```python
from build123d import *

# Parameters (mm, degrees)
F0_W          = 60.96
F0_H          = 91.44
F0_W_2        = 50.8
F0_H_2        = 86.614
F1_DEPTH      = 28.448
F3_DEPTH      = 25.4
F4_W          = 66.649839282
F4_H          = 6.9823637605
F5_DEPTH      = 3.048
F6_W          = 64.9686481762
F6_H          = 4.777956934
F7_DEPTH      = 3.048
F9_DEPTH      = 2.286
F10_W         = 99.848318845
F10_H         = 48.2080141082
F11_DEPTH     = 50.8
F13_T1_DEPTH  = 15.8581495789
F13_T3_DEPTH  = 15.8581495789
F13_T8_DEPTH  = 41.5121495789
F13_T13_DEPTH = 41.5121495789
F13_T18_DEPTH = 41.5121495789
F13_T23_DEPTH = 41.5121495789
F14_W         = 15.24
F14_H         = 23.368
F15_DEPTH     = 6.35
F16_W         = 5.3607832682
F16_H         = 13.1506472826
F17_DEPTH     = 25.909
F19_DEPTH     = 0.254
F20_DEPTH     = 0.254
F21_DEPTH     = 1.016
F22_W         = 3.175
F22_H         = 15.24
F22_H_2       = 15.425526537
F23_DEPTH     = 0.508
F24_W         = 3.175
F24_H         = 15.24
F24_H_2       = 15.1729788631
F25_DEPTH     = 0.508
F26_W         = 1.4869117904
F26_H         = 15.24
F26_H_2       = 15.1544166729
F27_DEPTH     = 0.508
F28_W         = 1.5113
F28_H         = 15.24
F28_W_2       = 1.492887156
F28_H_2       = 15.3870563954
F29_DEPTH     = 0.254
F30_DEPTH     = 0.381
F31_DEPTH     = 0.254
F32_W         = 105.9566885233
F32_H         = 116.2753328681
F33_DEPTH     = 14.5
F35_DEPTH     = 25
F36_DEPTH     = 1
F37_DEPTH     = 0.4
F38_DEPTH     = 0.4
F39_W         = 61.341
F39_H         = 89.424
F40_DEPTH     = 1.5
F41_T4_DEPTH  = 72.4640866379
F41_T9_DEPTH  = 72.4640866379


# Not quite as in the source:
# - a fillet or chamfer that OpenCascade refuses, or shapes differently, is made with other operations: its cross-section is extruded or revolved along the edge and cut away or added
# - a feature names something its author has since deleted; it is built from what else it names


with BuildPart() as f1:
    # F0 (on Top) → F1 (new body)
    with BuildSketch(Plane.XY):
        Rectangle(F0_W, F0_H)
        Rectangle(F0_W_2, F0_H_2, mode=Mode.SUBTRACT)
    extrude(amount=F1_DEPTH)

    # F2 (on face) → F3 (cut)
    with BuildSketch(Plane(origin=(0, 45.72, 0), x_dir=(-1, 0, 0), z_dir=(0, 1, 0))):
        Polygon((-9.4803553075, 0), (0, 0), (9.4803553075, 0), (5.461, 8.763), (-5.461, 8.763), align=None)
        Polygon((-9.4803553075, 28.448), (-5.461, 19.685), (5.461, 19.685), (9.4803553075, 28.448), (0, 28.448), align=None)
    extrude(amount=-F3_DEPTH, mode=Mode.SUBTRACT)

    # F4 (on Top) → F5 (cut)
    with BuildSketch(Plane.XY):
        with Locations((-0.1057945192, 44.6448102593)):
            Rectangle(F4_W, F4_H)
        with Locations((-0.1057945192, -44.6448102593)):
            Rectangle(F4_W, F4_H)
    extrude(amount=F5_DEPTH, mode=Mode.SUBTRACT)

    # F6 (on face) → F7 (cut)
    with BuildSketch(Plane.XY.offset(28.448)):
        with Locations((-2.0043240881, 43.331021533)):
            Rectangle(F6_W, F6_H)
        with Locations((-2.0043240881, -43.331021533)):
            Rectangle(F6_W, F6_H)
    extrude(amount=-F7_DEPTH, mode=Mode.SUBTRACT)

    # F8 (on face) → F9 (cut)
    with BuildSketch(Plane(origin=(25.4, 0, 0), x_dir=(0, -1, 0), z_dir=(-1, 0, 0))):
        Polygon((-43.0863499641, 0), (-41.1536283791, 0), (-25.9136283791, 0), (-25.9136283791, 30.48), (-41.1536283791, 30.48), (-43.0863499641, 30.48), align=None)
        Polygon((25.9136283791, 30.48), (25.9136283791, 0), (41.1536283791, 0), (43.0863499641, 0), (43.0863499641, 30.48), (41.1536283791, 30.48), align=None)
    extrude(amount=-F9_DEPTH, mode=Mode.SUBTRACT)

    # F10 (on Right) → F11 (cut)
    with BuildSketch(Plane.YZ):
        with Locations((1.7518345267, 13.4315635078)):
            Rectangle(F10_W, F10_H)
    extrude(amount=-F11_DEPTH, mode=Mode.SUBTRACT)

    # F12: F1 across plane


with BuildPart() as f1_1:
    add(f1.part)
    add(f1.part.mirror(Plane.YZ))

    # F13: chamfer of 2.54 on 12 edges, made by hand

    # F13_s2 → F13_t1 (cut)
    with BuildSketch(Plane.YZ.offset(-37.0120747894)):
        Polygon((38.402043066, 28.448), (40.942043066, 25.908), (40.942043066, 28.448), align=None)
        Polygon((38.6136283791, 0), (41.1536283791, 2.54), (41.1536283791, 0), align=None)
        Polygon((-40.942043066, 25.908), (-38.402043066, 28.448), (-40.942043066, 28.448), align=None)
        Polygon((-38.6136283791, 0), (-41.1536283791, 2.54), (-41.1536283791, 0), align=None)
    extrude(amount=F13_T1_DEPTH, mode=Mode.SUBTRACT)

    # F13_s4 → F13_t3 (cut)
    with BuildSketch(Plane.YZ.offset(21.1539252106)):
        Polygon((38.402043066, 28.448), (40.942043066, 25.908), (40.942043066, 28.448), align=None)
        Polygon((-40.942043066, 25.908), (-38.402043066, 28.448), (-40.942043066, 28.448), align=None)
        Polygon((-38.6136283791, 0), (-41.1536283791, 2.54), (-41.1536283791, 0), align=None)
        Polygon((38.6136283791, 0), (41.1536283791, 2.54), (41.1536283791, 0), align=None)
    extrude(amount=F13_T3_DEPTH, mode=Mode.SUBTRACT)


with BuildPart() as f13_tool6:
    # F13_s7 → F13_t8 (new body)
    with BuildSketch(Plane.XY.offset(-6.5320747894)):
        Polygon((25.4, 23.3736283791), (27.94, 25.9136283791), (25.4, 25.9136283791), align=None)
    extrude(amount=F13_T8_DEPTH)

    split(bisect_by=Plane.YZ.offset(27.686), keep=Keep.BOTTOM)


with BuildPart() as f1_2:
    add(f1_1.part)

    # F13_t5: cut F13_tool6
    add(f13_tool6.part, mode=Mode.SUBTRACT)


with BuildPart() as f13_tool11:
    # F13_s12 → F13_t13 (new body)
    with BuildSketch(Plane.XY.offset(34.9800747894)):
        Polygon((25.4, -23.3736283791), (27.94, -25.9136283791), (25.4, -25.9136283791), align=None)
    extrude(amount=-F13_T13_DEPTH)

    split(bisect_by=Plane.YZ.offset(27.686), keep=Keep.BOTTOM)


with BuildPart() as f1_3:
    add(f1_2.part)

    # F13_t10: cut F13_tool11
    add(f13_tool11.part, mode=Mode.SUBTRACT)


with BuildPart() as f13_tool16:
    # F13_s17 → F13_t18 (new body)
    with BuildSketch(Plane.XY.offset(-6.5320747894)):
        Polygon((-27.94, 25.9136283791), (-25.4, 23.3736283791), (-25.4, 25.9136283791), align=None)
    extrude(amount=F13_T18_DEPTH)

    split(bisect_by=Plane.YZ.offset(-27.686), keep=Keep.TOP)


with BuildPart() as f1_4:
    add(f1_3.part)

    # F13_t15: cut F13_tool16
    add(f13_tool16.part, mode=Mode.SUBTRACT)


with BuildPart() as f13_tool21:
    # F13_s22 → F13_t23 (new body)
    with BuildSketch(Plane.XY.offset(34.9800747894)):
        Polygon((-25.4, -23.3736283791), (-27.94, -25.9136283791), (-25.4, -25.9136283791), align=None)
    extrude(amount=-F13_T23_DEPTH)

    split(bisect_by=Plane.YZ.offset(-27.686), keep=Keep.TOP)


with BuildPart() as f1_5:
    add(f1_4.part)

    # F13_t20: cut F13_tool21
    add(f13_tool21.part, mode=Mode.SUBTRACT)

    # F14 (on face) → F15 (join)
    with BuildSketch(Plane.YZ.offset(30.48)):
        with Locations((-19.812, 14.224)):
            Rectangle(F14_W, F14_H)
        with Locations((19.812, 14.224)):
            Rectangle(F14_W, F14_H)
    extrude(amount=F15_DEPTH)

    # F16 (on face) → F17 (cut, through all)
    with BuildSketch(Plane.XY.offset(25.908)):
        with Locations((33.1603916341, -19.8066011071)):
            Rectangle(F16_W, F16_H)
        with Locations((33.1603916341, 19.8066011071)):
            Rectangle(F16_W, F16_H)
    extrude(amount=-F17_DEPTH, mode=Mode.SUBTRACT)

    # F18: F1 across plane


with BuildPart() as f1_6:
    add(f1_5.part)
    add(f1_5.part.mirror(Plane.YZ))

    # F19 (cut): faces of the model
    f19_faces = [f1_6.faces().sort_by_distance(p)[0] for p in [
        (26.543, -43.0863499641, 14.224),
        (-26.543, -43.0863499641, 14.224),
    ]]
    extrude(f19_faces, amount=-F19_DEPTH, mode=Mode.SUBTRACT)

    # F20 (cut): faces of the model
    f20_faces = [f1_6.faces().sort_by_distance(p)[0] for p in [
        (26.543, 43.0863499641, 14.224),
        (-26.543, 43.0863499641, 14.224),
    ]]
    extrude(f20_faces, amount=-F20_DEPTH, mode=Mode.SUBTRACT)

    # F21 (cut): a face of the model
    f21_faces = [f1_6.faces().sort_by_distance(p)[0] for p in [
        (0, -45.72, 14.224),
    ]]
    extrude(f21_faces, amount=-F21_DEPTH, mode=Mode.SUBTRACT)

    # F22 (on face) → F23 (join)
    with BuildSketch(Plane.XY.offset(25.908)):
        with Locations((-35.2425, 19.812)):
            Rectangle(F22_W, F22_H)
        with Locations((-35.2425, -19.7230628692)):
            Rectangle(F22_W, F22_H_2)
    extrude(amount=F23_DEPTH)

    # F24 (on face) → F25 (join)
    with BuildSketch(Plane(origin=(0, 0, 2.54), x_dir=(1, 0, 0), z_dir=(0, 0, -1))):
        with Locations((35.2425, 19.812)):
            Rectangle(F24_W, F24_H)
        with Locations((35.2425, -19.7903430089)):
            Rectangle(F24_W, F24_H_2)
    extrude(amount=F25_DEPTH)

    # F26 (on face) → F27 (join)
    with BuildSketch(Plane.XY.offset(25.908)):
        with Locations((36.0865441048, -19.812)):
            Rectangle(F26_W, F26_H)
        with Locations((36.0865441048, 19.7994005866)):
            Rectangle(F26_W, F26_H_2)
    extrude(amount=F27_DEPTH)

    # F28 (on face) → F29 (join)
    with BuildSketch(Plane(origin=(0, 0, 2.54), x_dir=(1, 0, 0), z_dir=(0, 0, -1))):
        with Locations((-36.07435, 19.812)):
            Rectangle(F28_W, F28_H)
        with Locations((-36.083556422, -19.7531366721)):
            Rectangle(F28_W_2, F28_H_2)
    extrude(amount=F29_DEPTH)

    # F30 (add): faces of the model
    f30_faces = [f1_6.faces().sort_by_distance(p)[0] for p in [
        (-30.48, 0.4258489378, 14.2172059936),
        (-35.3187, -19.812, 2.413),
        (-35.8407832682, -19.8066011071, 14.224),
        (-36.83, -19.8101053315, 14.3540262363),
    ]]
    extrude(f30_faces, amount=F30_DEPTH, dir=(-1, 0, 0))

    # F31 (add): a face of the model
    f31_faces = [f1_6.faces().sort_by_distance(p)[0] for p in [
        (-35.337112844, 19.7531366721, 2.413),
    ]]
    extrude(f31_faces, amount=F31_DEPTH)

    # F32 (on face) → F33 (cut)
    with BuildSketch(Plane.XY.offset(28.448)):
        with Locations((11.0789313912, -7.9427920282)):
            Rectangle(F32_W, F32_H)
    extrude(amount=-F33_DEPTH, mode=Mode.SUBTRACT)

    # F34 (on face) → F35 (join)
    with BuildSketch(Plane.XY.offset(13.948)):
        Polygon((-30.861, -27.432), (-30.861, -44.704), (30.48, -44.704), (30.48, -27.432), (30.48, -26.3819247484), (30.48, -13.2312774658), (30.48, -12.192), (30.48, 12.192), (30.48, 13.2312774658), (30.48, 26.3819247484), (30.48, 27.432), (30.48, 45.72), (-30.861, 45.72), (-30.861, 27.432), (-30.861, 26.3819247484), (-30.861, 13.2312774658), (-30.861, 12.192), (-30.861, -12.192), (-30.861, -13.2312774658), (-30.861, -26.3819247484), align=None)
        Polygon((-25.4, -43.3403499641), (-27.686, -43.3403499641), (-27.686, -25.6596283791), (-27.686, 25.6596283791), (-27.686, 43.3403499641), (-25.4, 43.3403499641), (25.4, 43.3403499641), (27.686, 43.3403499641), (27.686, 25.6596283791), (27.686, -25.6596283791), (27.686, -43.3403499641), (25.4, -43.3403499641), align=None, mode=Mode.SUBTRACT)
    extrude(amount=F35_DEPTH)

    # F36 (cut): a face of the model
    f36_faces = [f1_6.faces().sort_by_distance(p)[0] for p in [
        (-0.1974395314, 45.72, 21.5545051375),
    ]]
    extrude(f36_faces, amount=-F36_DEPTH, mode=Mode.SUBTRACT)

    # F37 (add): a face of the model
    f37_faces = [f1_6.faces().sort_by_distance(p)[0] for p in [
        (-35.083112844, 19.7531366721, 2.413),
    ]]
    extrude(f37_faces, amount=F37_DEPTH)

    # F38 (add): a face of the model
    f38_faces = [f1_6.faces().sort_by_distance(p)[0] for p in [
        (-35.3187, -19.812, 2.413),
    ]]
    extrude(f38_faces, amount=F38_DEPTH)

    # F39 (on face) → F40 (join)
    with BuildSketch(Plane.XY.offset(38.948)):
        with Locations((-0.1905, 0.008)):
            Rectangle(F39_W, F39_H)
    extrude(amount=F40_DEPTH)

    # F41: chamfer of 5 on 2 edges, made by hand


with BuildPart() as f41_tool2:
    # F41_s3 → F41_t4 (new body)
    with BuildSketch(Plane.XZ.offset(-36.2320433189)):
        Polygon((25.4, 8.948), (30.4, 13.948), (25.4, 13.948), align=None)
    extrude(amount=F41_T4_DEPTH)

    split(bisect_by=Plane.YZ.offset(27.686), keep=Keep.BOTTOM)


with BuildPart() as f1_7:
    add(f1_6.part)

    # F41_t1: cut F41_tool2
    add(f41_tool2.part, mode=Mode.SUBTRACT)


with BuildPart() as f41_tool7:
    # F41_s8 → F41_t9 (new body)
    with BuildSketch(Plane.XZ.offset(-36.2320433189)):
        Polygon((-25.4, 8.948), (-30.4, 13.948), (-25.4, 13.948), align=None)
    extrude(amount=F41_T9_DEPTH)

    split(bisect_by=Plane.YZ.offset(-27.686), keep=Keep.TOP)


with BuildPart() as f1_8:
    add(f1_7.part)

    # F41_t6: cut F41_tool7
    add(f41_tool7.part, mode=Mode.SUBTRACT)


solid = f1_8.part
```
For this review, take the finished solid that the model builds, in its own axes (mm). A direction names the side the tool comes from. Round coordinates to 2 decimals unless told otherwise and drop trailing zeros. Order: outer loops, then holes, each group sorted by start corner. A loop starts at its lowest first (then second) coordinate and runs counter-clockwise, first axis right, second up. Notation, with made-up numbers: (-17.75, 69.25) -> (19.25, 69.25) arc R15 cw to (19.25, 74.25) -> close; hole circle Ø1 at (66.5, 10.25). An arc over 180 degrees is marked (long way). Use a Markdown table: item, result.
Item 1: Draft analysis for pull direction X (two halves, no side actions). For faces 6 (the flat face through (-37.211, -20, 8)), 7 (the flat face through (-36, -20, 13.948)), 8 (the flat face through (33, -13.231, 8)), state which applies: +X half, -X half, draft (parallel to the pull), parting line (faces both ways), or undercut.
Resolved:
| item | result |
|---|---|
| face 6 | -X half |
| face 7 | draft |
| face 8 | undercut |
Item 2: For pin 1 (2.5 mm diameter, centred on x = 36, y = -20.5, fed in from -Z); pin 2 (5 mm diameter, centred on y = 30, z = 18, fed in from -X); pin 3 (1.5 mm diameter, centred on x = -12, y = -10.5, fed in from -Z), all flat-tipped, find the tip position at first contact; note any pin that passes through.
Resolved:
| item | result |
|---|---|
| pin 1 | stops at z = 2.03 |
| pin 2 | stops at x = -30.86 |
| pin 3 | stops at z = 38.95 |
Item 3: Take a section at C-C (y = 33). State the section outline as (x, z) points.
Resolved:
| item | result |
|---|---|
| outline | (-30.86, 0) -> (-27.69, 0) -> (-27.69, 38.95) -> (27.69, 38.95) -> (27.69, 0) -> (30.48, 0) -> (30.48, 40.45) -> (-30.86, 40.45) -> close |
Item 4: Machinability: for faces 1 (the flat face through (-36, 20, 13.948)), 2 (the flat face through (19, 44, 3.048)), 3 (the flat face through (-33, -13.231, 8)), 4 (the flat face through (34, -27.432, 8)), 5 (the flat face through (35, -20, 2.032)), which of the approach directions +Z, -Z, +X, -X, +Y, -Y give a long, thin tool a straight path to every point of the face, cutting with its end or side? Answer none if there is none.
Resolved:
| item | result |
|---|---|
| face 1 | +Z, -X, +Y, -Y |
| face 2 | -Z, +X, -X, +Y |
| face 3 | +Z |
| face 4 | +Z, -Z, +X, -Y |
| face 5 | -Z, +X, +Y, -Y |
Item 5: Take a section at A-A (y = 15). State the section outline as (x, z) points (3 decimals), plus the area to 3 significant figures.
Resolved:
| item | result |
|---|---|
| outline | (-36.83, 2.286) -> (-34.683, 2.286) -> (-34.683, 2.54) -> (-35.841, 2.54) -> (-35.841, 13.948) -> (-36.83, 13.948) -> close; (-30.861, 0) -> (-25.4, 0) -> (-25.4, 8.948) -> (-27.686, 11.234) -> (-27.686, 38.948) -> (27.686, 38.948) -> (27.686, 11.234) -> (25.4, 8.948) -> (25.4, 0) -> (30.48, 0) -> (30.48, 40.448) -> (-30.861, 40.448) -> close; (33.655, 2.032) -> (36.83, 2.032) -> (36.83, 13.948) -> (35.841, 13.948) -> (35.841, 2.54) -> (33.655, 2.54) -> close |
| area | 395 mm² |
Item 6: Take a section at D-D (z = 26). State the section outline as (x, y) points, plus the area to 3 significant figures.
Resolved:
| item | result |
|---|---|
| outline | (-30.86, -44.7) -> (30.48, -44.7) -> (30.48, 44.72) -> (-30.86, 44.72) -> close; hole (-27.69, -43.34) -> (27.69, -43.34) -> (27.69, 43.34) -> (-27.69, 43.34) -> close |
| area | 686 mm² |
Item 7: For line 1 along X through (y, z) = (18, 11.5); line 2 along Y through (x, z) = (-26.5, 15); line 3 along X through (y, z) = (3, 19), list the stretches that pass through material, from the lowest coordinate up. Write a range as [from, to].
Resolved:
| item | result |
|---|---|
| line 1 | x = [-36.83, -35.84], [-30.86, -27.69], [27.69, 30.48], [35.84, 36.83] |
| line 2 | y = [-44.7, -43.34], [43.34, 44.72] |
| line 3 | x = [-30.86, -27.69], [27.69, 30.48] |
